```python
from build123d import *

# Parameters (mm, degrees)
CUT_EXTRUDE1_REACH = 25.971
SKETCH16_R         = 6.477
CHAMFER1_SIZE      = 0.635


with BuildPart() as part:
    # Sketch1 → Revolve1 (revolve)
    with BuildSketch(Plane(origin=(0, 0, 0), x_dir=(0, 0, -1), z_dir=(1, 0, 0)), mode=Mode.PRIVATE) as revolve1_sk:
        Polygon((0, 0), (0, 12.7), (3.175, 12.7), (3.175, 9.525), (15.875, 9.525), (15.875, 0), align=None)
    revolve(revolve1_sk.sketch.rotate(Axis((0, 0, 0), (0, 0, 1)), 90), axis=Axis((0, 0, 0), (0, 0, 1)))

    # Sketch16 → Cut-Extrude1 (cut, up to next)
    with BuildSketch(Plane.XY, mode=Mode.PRIVATE) as cut_extrude1_sk1:
        Circle(SKETCH16_R)
    cut_extrude1_tool1 = extrude(cut_extrude1_sk1.sketch, amount=-CUT_EXTRUDE1_REACH, mode=Mode.PRIVATE) & part.part
    add(cut_extrude1_tool1.solids().sort_by_distance((0, 0, 0))[0], mode=Mode.SUBTRACT)

    # Chamfer1
    chamfer1_edges = [part.edges().sort_by_distance(p)[0] for p in [
        (-6.477, 0, -15.875),
        (-6.477, 0, 0),
        (9.525, 0, -15.875),
        (9.525, 0, -3.175),
        (12.7, 0, -3.175),
        (12.7, 0, 0),
    ]]
    chamfer(chamfer1_edges, length=CHAMFER1_SIZE)


solid = part.part
```
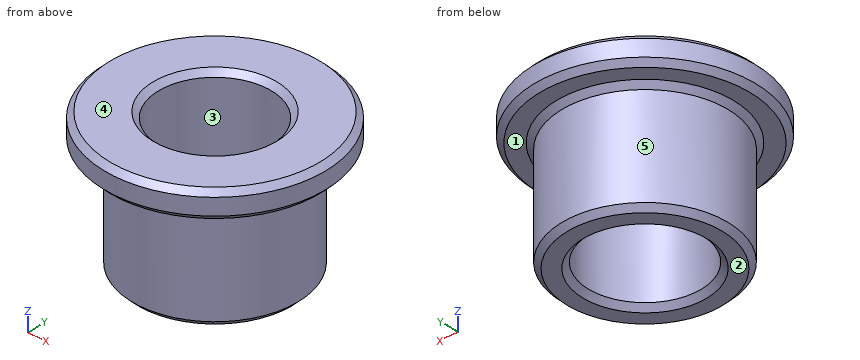
Read the model definition and answer for the solid it produces. Units are mm, in the model's axes. Face numbers are marked on the shaded views. A direction names the side the tool comes from. Coordinates: 2 decimals unless noted, no trailing zeros. Loops run counter-clockwise (first coordinate to the right, second up) from the corner with the lowest first, then second, coordinate; pieces in that order, holes last. Notation, with made-up numbers: (54, 25.25) - (67, 25.25) arc R21 ccw to (67, 42.25) - close; hole circle Ø9 at (64, 61.5). An arc over 180 degrees is marked (long way). Answer in a Markdown table with one row per item.
1. Find section A-A, the plane y = 0. Write down the section's boundary in (x, z) (3 decimals).
Conclusion:
| item | result |
|---|---|
| outline | (-12.7, -2.54) - (-12.065, -3.175) - (-10.16, -3.175) - (-9.525, -3.81) - (-9.525, -15.24) - (-8.89, -15.875) - (-7.112, -15.875) - (-6.477, -15.24) - (-6.477, -0.635) - (-7.112, 0) - (-12.065, 0) - (-12.7, -0.635) - close; (6.477, -15.24) - (7.112, -15.875) - (8.89, -15.875) - (9.525, -15.24) - (9.525, -3.81) - (10.16, -3.175) - (12.065, -3.175) - (12.7, -2.54) - (12.7, -0.635) - (12.065, 0) - (7.112, 0) - (6.477, -0.635) - close |
2. Which of the six approach directions +Z, -Z, +X, -X, +Y, -Y give full straight-line access (tool end or side, diameter ignored) to the marked faces 1 and 2?
Conclusion:
| item | result |
|---|---|
| face 1 | -Z |
| face 2 | -Z, +X, -X, +Y, -Y |
3. Given pin 1 (2 mm diameter, centred on x = 3, z = -2, fed in from +Y); pin 2 (2 mm diameter, centred on x = -4, z = -1.5, fed in from +Y); pin 3 (3 mm diameter, centred on y = -6, z = -10.5, fed in from -X) (3 decimals), each flat-ended and moving along its own axis, determine where each tip first touches the part or whether it passes through.
Conclusion:
| item | result |
|---|---|
| pin 1 | stops at y = 12.54 |
| pin 2 | stops at y = 12.34 |
| pin 3 | stops at x = -8.395 |
4. Straight lines are drawn through the part: line 1 (Y direction, x = 0, z = -4.75) (3 decimals); line 2 (Y direction, x = -3.25, z = -5.5); line 3 (X direction, y = 4.75, z = -5.5). For each, find the intervals that lie inside material, in ascending order.
Conclusion:
| item | result |
|---|---|
| line 1 | y = -9.525 to -6.477, 6.477 to 9.525 |
| line 2 | y = -8.95 to -5.6, 5.6 to 8.95 |
| line 3 | x = -8.26 to -4.4, 4.4 to 8.26 |
5. Find section C-C, the plane z = -4.5. Write down the section's boundary in (x, y) (3 decimals), then the cut area to 3 significant figures.
Conclusion:
| item | result |
|---|---|
| outline | circle Ø19.05 at (0, 0); hole circle Ø12.954 at (0, 0) |
| area | 153 mm² |
6. Determine the mould class of the marked faces 3, 4 and 5 for opening direction X: +X half, -X half, draft (parallel to the pull), parting line (faces both ways), or undercut.
Conclusion:
| item | result |
|---|---|
| face 3 | undercut |
| face 4 | draft |
| face 5 | parting line |
